Autodesk Inventor part; units mm, degrees
ref_plane "Work Plane1" through (7, 0, -2.75) normal (0, 0, 1) x (1, 0, 0)
ref_plane "YZ Plane" through (0, 0, 0) normal (1, 0, 0) x (0, 1, 0)
ref_plane "XZ Plane" through (0, 0, 0) normal (0, 1, 0) x (-1, 0, 0)
sketch "Sketch1" plane through (0, 0, 0) normal (0, 1, 0) x (-1, 0, 0)
  line L0 (5, 0) -> (16.619, -3)
  line L1 (5, 0) -> (-7, 0)
  arc A0 (-7, 0) -> (16.619, -3) centre (5, 0) ccw
  line L2 (0, 0) -> (-12, 0)
  arc A1 (-14, 0) -> (23.3548, -4.9094) centre (5, 0) ccw
  line L3 (16.619, -3) -> (23.3548, -4.9094)
  line L4 (-7, 0) -> (-14, 0)
  point P0 (-7, 0)
  dimension "d0" = 12
  dimension "d2" = 3
  dimension "d3" = 12
  dimension "d4" = 0
  dimension "d5" = 5
  dimension "d6" = 0
  dimension "d7" = 7
extrude "Extrusion1" add sketch "Sketch1" along normal blind 10 contours L3 A1 L4 L2 A0
ref_plane "Work Plane1" through (7, 0, -2.75) normal (0, 0, 1) x (1, 0, 0)
split "Split1" plane through (7, 0, -2.75) removes the side toward (0, 0, 1)
sketch "Sketch2" plane through (6.6806, 0, -2.75) normal (0, 0, 1) x (1, 0, 0)
  line L0 (0, 0) -> (0, 10)
  line L1 (7.1193, 0) -> (0, 0)
  line L2 (7.1193, 10) -> (7.1193, 0)
  line L3 (0, 10) -> (7.1193, 10)
  point P0 (-6.6806, 0)
extrude "Extrusion2" add sketch "Sketch2" along normal blind 5.5
sketch "Sketch3" plane through (13.7999, 0, -2.75) normal (1, 0, 0) x (0, 0, -1)
  line L0 (0, 10) -> (0, 0)
  line L1 (0, 10) -> (-5.5, 10)
  line L2 (-5.5, 0) -> (-5.5, 10)
  line L3 (0, 0) -> (-5.5, 0)
  point P0 (-2.75, 0)
extrude "Extrusion3" add sketch "Sketch3" along normal blind 10
sketch "Sketch4" plane through (0, 0, 0) normal (0, -1, 0) x (1, 0, 0)
  line L0 (6.6806, -2.75) -> (6.6806, 2.75)
  point P0 (0, 0)
  point P1 (10.2403, 0)
  point P2 (13.7999, -2.75)
  dimension "d15" = 0
  dimension "d16" = 3.5596
  dimension "d17" = 7.1193
hole "Hole1" at (10.2403, 0, 0) direction (0, 1, 0) diameter 3.25 end through all
sketch "Sketch5" plane through (6.6806, 0, -2.75) normal (-1, 0, 0) x (0, 0, 1)
  line L0 (5.5, 0) -> (-6.5, 0)
  line L1 (-6.5, 0) -> (-6.5, 5.25)
  line L2 (-6.5, 5.25) -> (5.5, 5.25)
  line L3 (5.5, 5.25) -> (5.5, 0)
  line L4 (0, 12) -> (0, -2)
  dimension "d29" = 5.25
  dimension "d30" = 6.5
extrude "halfCut" cut sketch "Sketch5" along normal blind 5.5 and the other way blind 20
fillet "Fillet1" radius 1 1 edges at (7.1204, 5.25, -9.25)
sketch "Sketch6" plane through (6.6806, 0, 2.75) normal (0, 0, 1) x (1, 0, 0)
  line L0 (0, 10) -> (17.1193, 10)
  line L1 (0, 5.25) -> (17.1193, 5.25)
  line L2 (17.1193, 10) -> (17.1193, 5.25)
  point P0 (-6.6806, 0)
  point P1 (14.6193, 7.625)
  dimension "d33" = 2.375
  dimension "d34" = 4.75
  dimension "d35" = 2.5
hole "Hole2" at (21.2999, 7.625, 2.75) direction (0, 0, -1) diameter 2 end through all
equation "\"d0\" = r"
equation "\"d2\" = 0.5 * a1"
equation "\"d3\" = r"
equation "\"d7\" = t"
equation "\"d11\" = a2"
equation "\"d18\" = dpin"
equation "\"d28\" = fillet"
equation "\"d36\" = dcable"
equation "\"r\" = 12"
equation "\"t\" = 7"
equation "\"a1\" = 6"
equation "\"a2\" = 5.5"
equation "\"d10\" = -0.5 * a2"
equation "\"dpin\" = 3.25"
equation "\"fillet\" = 1"
equation "\"dcable\" = 2"
properties part number "holder2_clamp" material "Steel, Mild"
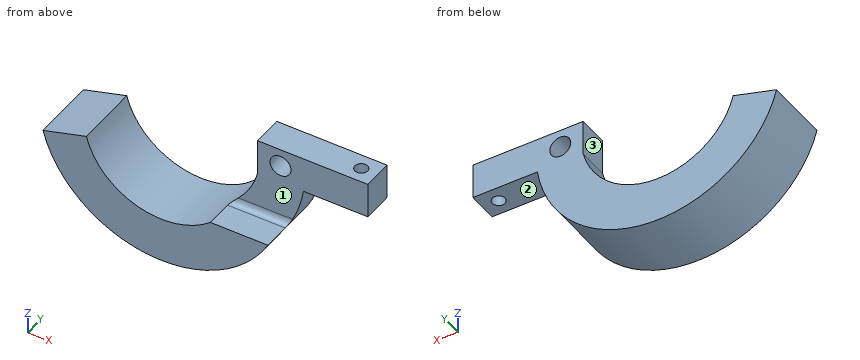
Geometry check sheet. Reference: the model listing, model coordinates, mm. Face numbers are marked on the shaded views. A direction names the side the tool comes from. Give positions to 0.01 mm unless a question says otherwise; leave off trailing zeros. Order: outer loops, then holes, each group sorted by start corner. A loop starts at its lowest first (then second) coordinate and runs counter-clockwise, first axis right, second up. Notation, with made-up numbers: M -0.75,-40 L 24.25,-40 A16 cw 24.25,-19 Z; hole C -26,-2 d4. An arc over 180 degrees is marked long. Use a Markdown table: item, result.
Item 1: Material ranges on line 1 along Z through (x, y) = (-4.5, 1.25); line 2 along X through (y, z) = (7.25, 0); line 3 along Z through (x, y) = (17.5, 8.75), recorded low to high.
Answers follow:
| item | result |
|---|---|
| line 1 | z = -18.99 to -11.99 |
| line 2 | x = 6.68 to 8.62, 11.87 to 20.37, 22.23 to 23.8 |
| line 3 | z = -2.75 to 2.75 |
Item 2: Section check D-D (x = 5). Record the cut outline in (y, z).
Answers follow:
| item | result |
|---|---|
| outline | M 0,-16.16 L 10,-16.16 L 10,-6.63 L 5.25,-6.63 L 5.25,-8.25 A1 cw 4.25,-9.25 L 0,-9.25 Z |
Item 3: Tool access check on the marked faces 1, 2 and 3. Record the directions out of +Z, -Z, +X, -X, +Y, -Y that give a thin tool (end or side, any length) a straight path to the whole face; none if there is none.
Answers follow:
| item | result |
|---|---|
| face 1 | +Z, +X, -Y |
| face 2 | -Z, +X, +Y, -Y |
| face 3 | +Z, -X, +Y, -Y |
Item 4: Depth check by flat-ended pin: P1, Ø4, axis at x = 16.5, y = 7, coming from the -Z side; P2, Ø3, axis at y = 4, z = -12.5, coming from the +X side; P3, Ø2.5, axis at y = 8.5, z = -0.5, coming from the -X side. Enter the tip coordinate at first touch or a pass-through.
Answers follow:
| item | result |
|---|---|
| P1 | stops at z = -2.75 |
| P2 | stops at x = 10.49 |
| P3 | stops at x = 6.68 |
Item 5: Section check A-A (z = 0). Record the cut outline in (x, y) (3 decimals), and give its area (3 significant figures).
Answers follow:
| item | result |
|---|---|
| outline | M 6.681,5.25 L 8.615,5.25 L 8.615,10 L 6.681,10 Z; M 11.865,5.25 L 23.8,5.25 L 23.8,10 L 11.865,10 Z; hole C 21.3,7.625 d2 |
| area | 62.7 mm2 |
Item 6: Section check B-B (z = -10). Record the cut outline in (x, y).
Answers follow:
| item | result |
|---|---|
| outline | M -21.16,0 L -11.63,0 L -11.63,10 L -21.16,10 Z; M 1.63,0 L 11.16,0 L 11.16,10 L 1.63,10 Z |
